Read the model definition and answer for the solid it produces. Units are mm, in the model's axes. Face numbers are marked on the shaded views. Round coordinates to 2 decimals unless told otherwise and drop trailing zeros. Order: outer loops, then holes, each group sorted by start corner. A loop starts at its lowest first (then second) coordinate and runs counter-clockwise, first axis right, second up. Notation, with made-up numbers: (18.25, -5) - (51.25, -5) arc R9 cw to (51.25, 8) - close; hole circle Ø4 at (8, -21). An arc over 180 degrees is marked (long way). Answer as a JSON object with one key per item and string values. Group by question number.
Q1. A cutting plane is placed at A-A on x = 0. Determine the outline of the cut face in (y, z), and give its area (3 significant figures).
Q2. Consider line 1 (Y direction, x = 0, z = 8); line 2 (Z direction, x = 0, y = -19); line 3 (Z direction, x = 12.5, y = 7.5). Determine where each line is inside the solid, lowest interval first.
Q3. The mould has two halves that part along X. Classify the marked faces 1, 2, 3 and 4: pulls with the +X half, pulls with the -X half, needs draft (parallel to the pull), parting line crosses it, or undercut.
Q4. Given pin 1 Ø2 at (x, z) = (18.5, 13) entering from -Y; pin 2 Ø12 at (x, y) = (-5, -9) entering from -Z; pin 3 Ø6 at (y, z) = (5, 21.5) entering from +X, each flat-ended and moving along its own axis, determine where each tip first touches the part or whether it passes through.
Q5. A cutting plane is placed at B-B on z = 15. Determine the outline of the cut face in (x, y).
Q6. A cutting plane is placed at C-C on z = 22.5. Determine the outline of the cut face in (x, y), and give its area (3 significant figures).
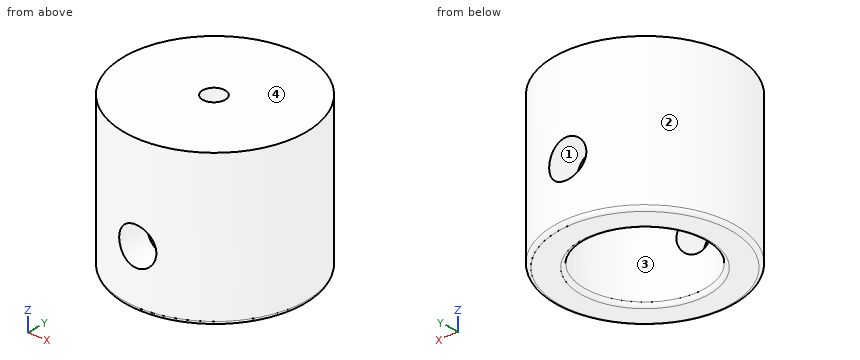
```python
from build123d import *

# Parameters (mm, degrees)
F0_R      = 24
F1_DEPTH  = 40
F2_R      = 16
F3_DEPTH  = 25
F4_R      = 3
F5_DEPTH  = 25
F6_R      = 0.2
F7_R      = 1
F8_R      = 5
F9_DEPTH  = 50
F10_R     = 5
F11_DEPTH = 25


with BuildPart() as f1:
    # F0 (on Top) → F1 (new body)
    with BuildSketch(Plane.XY):
        Circle(F0_R)
    extrude(amount=F1_DEPTH)

    # F2 (on face) → F3 (cut)
    with BuildSketch(Plane(origin=(0, 0, 0), x_dir=(1, 0, 0), z_dir=(0, 0, -1))):
        Circle(F2_R)
    extrude(amount=-F3_DEPTH, mode=Mode.SUBTRACT)

    # F4 (on face) → F5 (cut)
    with BuildSketch(Plane(origin=(0, 0, 25), x_dir=(1, 0, 0), z_dir=(0, 0, -1))):
        with Locations((0, 0.3276021098)):
            Circle(F4_R)
    extrude(amount=-F5_DEPTH, mode=Mode.SUBTRACT)

    # F6
    f6_edges = [f1.edges().sort_by_distance(p)[0] for p in [
        (-3, -0.327602, 25),
        (-16, 0, 25),
    ]]
    fillet(f6_edges, radius=F6_R)

    # F7
    f7_edges = [f1.edges().sort_by_distance(p)[0] for p in [
        (-16, 0, 0),
        (-24, 0, 0),
    ]]
    fillet(f7_edges, radius=F7_R)

    # F8 (on Front) → F9 (cut)
    with BuildSketch(Plane.XZ):
        with Locations((0, 15)):
            Circle(F8_R)
    extrude(amount=F9_DEPTH, mode=Mode.SUBTRACT)

    # F10 (on Front) → F11 (cut)
    with BuildSketch(Plane.XZ):
        with Locations((0, 15)):
            Circle(F10_R)
    extrude(amount=-F11_DEPTH, mode=Mode.SUBTRACT)


solid = f1.part
```
Result set:
{
 "1": {"outline": "(-24, 1) arc R1 ccw to (-23, 0) - (-17, 0) arc R1 ccw to (-16, 1) - (-16, 10) - (-24, 10) - close; (-24, 20) - (-16, 20) - (-16, 24.8) arc R0.2 cw to (-15.8, 25) - (-3.53, 25) arc R0.2 ccw to (-3.33, 25.2) - (-3.33, 40) - (-24, 40) - close; (2.67, 25.2) arc R0.2 ccw to (2.87, 25) - (15.8, 25) arc R0.2 cw to (16, 24.8) - (16, 20) - (24, 20) - (24, 40) - (2.67, 40) - close; (16, 1) arc R1 ccw to (17, 0) - (23, 0) arc R1 ccw to (24, 1) - (24, 10) - (16, 10) - close", "area": "869 mm²"},
 "2": {"line 1": "y = -24 to -16, 16 to 24", "line 2": "z = 0 to 10, 20 to 40", "line 3": "z = 25 to 40"},
 "3": {"face 1": "undercut", "face 2": "parting line crosses it", "face 3": "undercut", "face 4": "needs draft"},
 "4": {"pin 1": "stops at y = -16.42", "pin 2": "stops at z = 0.29", "pin 3": "stops at x = 23.92"},
 "5": {"outline": "(-5, -23.47) - (-5, -15.2) arc R16 cw to (-5, 15.2) - (-5, 23.47) arc R24 ccw to start; (5, -23.47) arc R24 ccw to (5, 23.47) - (5, 15.2) arc R16 cw to (5, -15.2) - close"},
 "6": {"outline": "circle Ø48 at (0, 0); hole circle Ø32 at (0, 0)", "area": "1,010 mm²"}
}
